from build123d import *

# Parameters (mm, degrees)
BOSS_EXTRUDE1_DEPTH = 2.54
SKETCH3_R           = 2.54
BOSS_EXTRUDE2_DEPTH = 2.54
SKETCH4_R           = 1.143
CUT_EXTRUDE1_DEPTH  = 152.042782279
SKETCH5_R           = 1.858808724
SKETCH5_R_2         = 1.906231368
CUT_EXTRUDE2_DEPTH  = 151.978698095


with BuildPart() as part:
    # Sketch2 → Boss-Extrude1 (new body)
    with BuildSketch(Plane.XY):
        with BuildLine():
            Line((-114.427, 27.932368959), (-120.015, 27.932368959))
            Line((-120.015, 27.932368959), (-120.015, 42.483412464))
            Line((-120.015, 42.483412464), (-82.806810404, 42.483412464))
            Line((-82.806810404, 42.483412464), (-82.801193697, 35.552368959))
            Line((-82.801193697, 35.552368959), (-12.708278928, 35.552368959))
            Line((-12.708278928, 35.552368959), (-12.713937882, 42.544153403))
            Line((-12.713937882, 42.544153403), (12.708274756, 42.545846409))
            Line((12.708274756, 42.545846409), (12.708274756, -33.146999807))
            Line((12.708274756, -33.146999807), (12.708274756, -91.058999807))
            Line((12.708274756, -91.058999807), (5.088274756, -91.058999807))
            Line((5.088274756, -91.058999807), (5.088274756, -78.358999807))
            ThreePointArc((5.088274756, -78.358999807), (1.368530877, -69.378743686), (-7.611725244, -65.658999807))
            Line((-7.611725244, -65.658999807), (-61.849, -65.658999807))
            ThreePointArc((-61.849, -65.658999807), (-70.829256121, -69.378743686), (-74.549, -78.358999807))
            Line((-74.549, -78.358999807), (-74.549, -85.724999807))
            Line((-74.549, -85.724999807), (-74.549, -91.566999807))
            Line((-74.549, -91.566999807), (-82.169, -91.566999807))
            Line((-82.169, -91.566999807), (-82.169, -85.724999807))
            Line((-82.169, -85.724999807), (-82.169, -78.358999807))
            ThreePointArc((-82.169, -78.358999807), (-85.888743879, -69.378743686), (-94.869, -65.658999807))
            Line((-94.869, -65.658999807), (-120.015, -65.658999807))
            Line((-120.015, -65.658999807), (-120.015, -45.846999807))
            Line((-120.015, -45.846999807), (-114.427, -45.846999807))
            Line((-114.427, -45.846999807), (-114.427, 27.932368959))
        make_face()
    extrude(amount=BOSS_EXTRUDE1_DEPTH)

    # Sketch3 → Boss-Extrude2 (add)
    with BuildSketch(Plane.XY.offset(2.54)):
        with Locations((-63.432362622, -59.308999807)):
            Circle(SKETCH3_R)
        with Locations((-6.028362622, -59.308999807)):
            Circle(SKETCH3_R)
        with Locations((-6.028362622, -11.048999807)):
            Circle(SKETCH3_R)
        with Locations((-63.432362622, -11.048999807)):
            Circle(SKETCH3_R)
    extrude(amount=BOSS_EXTRUDE2_DEPTH)

    # Sketch4 → Cut-Extrude1 (cut, through all)
    with BuildSketch(Plane.XY.offset(5.08)):
        with Locations((-6.028362622, -59.308999807)):
            Circle(SKETCH4_R)
        with Locations((-63.432362622, -59.308999807)):
            Circle(SKETCH4_R)
        with Locations((-63.432362622, -11.048999807)):
            Circle(SKETCH4_R)
        with Locations((-6.028362622, -11.048999807)):
            Circle(SKETCH4_R)
    extrude(amount=-CUT_EXTRUDE1_DEPTH, mode=Mode.SUBTRACT)

    # Sketch5 → Cut-Extrude2 (cut, through all)
    with BuildSketch(Plane.XY.offset(2.54)):
        with Locations((-8.811927589, 15.209269476)):
            Circle(SKETCH5_R)
        with Locations((-49.660967681, 15.209269476)):
            Circle(SKETCH5_R_2)
    extrude(amount=-CUT_EXTRUDE2_DEPTH, mode=Mode.SUBTRACT)


solid = part.part
The model under review builds one solid part; all positions refer to its coordinate system, in mm. A direction names the side the tool comes from. Round coordinates to 2 decimals unless told otherwise and drop trailing zeros. Write each loop counter-clockwise with the first axis right and the second up, starting at its lowest first coordinate (ties: lowest second). Pieces come first, ordered by that corner, then holes. Notation, with made-up numbers: (-16, -25.5) - (-1, -25.5) arc R33 ccw to (-1, 5.5) - close; hole circle Ø10 at (-23, 25.25). An arc over 180 degrees is marked (long way). One line per item, written item: value. Start each with the question number.
1. Consider section A-A on y = -82.5. Write out the cut boundary in (x, z), and give its area (3 significant figures).
2. Consider section B-B on z = 1.3. Write out the cut boundary in (x, y) (3 decimals).
3. Machinability: for faces 1 (the face through (1.47, -69.48, 1.25)), 2 (the face through (-6.58, -61.79, 3.79)), 3 (the face through (-6, -58, 5.08)), which of the approach directions +Z, -Z, +X, -X, +Y, -Y give a long, thin tool a straight path to every point of the face, cutting with its end or side? Answer none if there is none.
4. Clearance check with flat-ended pins moving along their axes: P1, Ø1.3, axis at x = -53, z = 1.5, coming from the +Y side; P2, Ø0.8, axis at y = -87.5, z = 1.5, coming from the -X side; P3, Ø2, axis at x = 9.5, z = 1.5, coming from the -Y side. State where each tip first meets the part, or that it passes through.
5. The part is to be moulded in two halves that separate along Y. For faces 4 (the face through (-5, -12, 5.08)), 5 (the face through (-70.73, -69.28, 1.25)), 6 (the face through (-9.054, 17.052, 1.288)), say which applies: released by +Y, released by -Y, zero draft, split by the parting line, or undercut.
6. Consider section D-D on x = -101.5. Write out the cut boundary in (y, z).
7. To check wall thickness, follow L1, parallel to X at y = -59, z = 1.95 (3 decimals); L2, parallel to X at y = 25, z = 2.05; L3, parallel to Y at x = -30, z = 0.5. State the ranges of each line that lie inside material, in increasing order. Write a range as from..to.
8. Consider section C-C on y = 31. Write out the cut boundary in (x, z) (3 decimals).
Checks:
1. outline: (-82.17, 0) - (-74.55, 0) - (-74.55, 2.54) - (-82.17, 2.54) - close; (5.09, 0) - (12.71, 0) - (12.71, 2.54) - (5.09, 2.54) - close
1. area: 38.7 mm^2
2. outline: (-120.015, -65.659) - (-94.869, -65.659) arc R12.7 cw to (-82.169, -78.359) - (-82.169, -91.567) - (-74.549, -91.567) - (-74.549, -78.359) arc R12.7 cw to (-61.849, -65.659) - (-7.612, -65.659) arc R12.7 cw to (5.088, -78.359) - (5.088, -91.059) - (12.708, -91.059) - (12.708, 42.546) - (-12.714, 42.544) - (-12.708, 35.552) - (-82.801, 35.552) - (-82.807, 42.483) - (-120.015, 42.483) - (-120.015, 27.932) - (-114.427, 27.932) - (-114.427, -45.847) - (-120.015, -45.847) - close; hole circle Ø2.286 at (-63.432, -59.309); hole circle Ø2.286 at (-63.432, -11.049); hole circle Ø3.812 at (-49.661, 15.209); hole circle Ø3.718 at (-8.812, 15.209); hole circle Ø2.286 at (-6.028, -59.309); hole circle Ø2.286 at (-6.028, -11.049)
3. face 1: +Z, -Z, -Y
3. face 2: +Z
3. face 3: +Z, +X, -X, +Y, -Y
4. P1: stops at y = 35.55
4. P2: stops at x = -82.17
4. P3: stops at y = -91.06
5. face 4: zero draft
5. face 5: released by -Y
5. face 6: undercut
6. outline: (-65.66, 0) - (42.48, 0) - (42.48, 2.54) - (-65.66, 2.54) - close
7. L1: x = -120.015..-64.533, -62.332..-7.129, -4.928..12.708
7. L2: x = -114.43..12.71
7. L3: y = -65.66..35.55
8. outline: (-120.015, 0) - (12.708, 0) - (12.708, 2.54) - (-120.015, 2.54) - close
